from build123d import *

# Parameters (mm, degrees)
SKETCH1_R           = 2.1
SKETCH1_R_2         = 13
BOSS_EXTRUDE1_DEPTH = 0.4
BOSS_EXTRUDE2_DEPTH = 0.4


with BuildPart() as part:
    # Sketch1 → Boss-Extrude1 (new body)
    with BuildSketch(Plane(origin=(0, 0, 0), x_dir=(0, 1, 0), z_dir=(0, 0, 1))):
        with BuildLine():
            ThreePointArc((21.242857143, -3.31527079), (21.435617889, -1.662614121), (21.5, 0))
            ThreePointArc((21.5, 0), (21.435617889, 1.662614121), (21.242857143, 3.31527079))
            ThreePointArc((21.242857143, 3.31527079), (19.220493395, 4.694667451), (16.785714286, 4.948716593))
            ThreePointArc((16.785714286, 4.948716593), (12.374368671, 12.374368671), (4.948716593, 16.785714286))
            ThreePointArc((4.948716593, 16.785714286), (4.694667451, 19.220493395), (3.31527079, 21.242857143))
            ThreePointArc((3.31527079, 21.242857143), (0, 21.5), (-3.31527079, 21.242857143))
            ThreePointArc((-3.31527079, 21.242857143), (-4.694667451, 19.220493395), (-4.948716593, 16.785714286))
            ThreePointArc((-4.948716593, 16.785714286), (-12.374368671, 12.374368671), (-16.785714286, 4.948716593))
            ThreePointArc((-16.785714286, 4.948716593), (-19.220493395, 4.694667451), (-21.242857143, 3.31527079))
            ThreePointArc((-21.242857143, 3.31527079), (-21.5, 0), (-21.242857143, -3.31527079))
            ThreePointArc((-21.242857143, -3.31527079), (-19.220493395, -4.694667451), (-16.785714286, -4.948716593))
            ThreePointArc((-16.785714286, -4.948716593), (-12.374368671, -12.374368671), (-4.948716593, -16.785714286))
            ThreePointArc((-4.948716593, -16.785714286), (-4.694667451, -19.220493395), (-3.31527079, -21.242857143))
            ThreePointArc((-3.31527079, -21.242857143), (0, -21.5), (3.31527079, -21.242857143))
            ThreePointArc((3.31527079, -21.242857143), (4.694667451, -19.220493395), (4.948716593, -16.785714286))
            ThreePointArc((4.948716593, -16.785714286), (12.374368671, -12.374368671), (16.785714286, -4.948716593))
            ThreePointArc((16.785714286, -4.948716593), (19.220493395, -4.694667451), (21.242857143, -3.31527079))
        make_face()
        with Locations((0, -17.5)):
            Circle(SKETCH1_R, mode=Mode.SUBTRACT)
        Circle(SKETCH1_R_2, mode=Mode.SUBTRACT)
        with Locations((17.5, 0)):
            Circle(SKETCH1_R, mode=Mode.SUBTRACT)
        with Locations((-17.5, 0)):
            Circle(SKETCH1_R, mode=Mode.SUBTRACT)
        with Locations((0, 17.5)):
            Circle(SKETCH1_R, mode=Mode.SUBTRACT)
    extrude(amount=BOSS_EXTRUDE1_DEPTH)

    # Sketch1_4 → Boss-Extrude2 (add)
    with BuildSketch(Plane(origin=(0, 0, 0), x_dir=(0, 1, 0), z_dir=(0, 0, 1))):
        with BuildLine():
            ThreePointArc((-21.242857143, -3.31527079), (-15.202795796, -15.202795796), (-3.31527079, -21.242857143))
            ThreePointArc((-3.31527079, -21.242857143), (-4.694667451, -19.220493395), (-4.948716593, -16.785714286))
            ThreePointArc((-4.948716593, -16.785714286), (-12.374368671, -12.374368671), (-16.785714286, -4.948716593))
            ThreePointArc((-16.785714286, -4.948716593), (-19.220493395, -4.694667451), (-21.242857143, -3.31527079))
        make_face()
        with BuildLine():
            ThreePointArc((-4.948716593, 16.785714286), (-4.694667451, 19.220493395), (-3.31527079, 21.242857143))
            ThreePointArc((-3.31527079, 21.242857143), (-15.202795796, 15.202795796), (-21.242857143, 3.31527079))
            ThreePointArc((-21.242857143, 3.31527079), (-19.220493395, 4.694667451), (-16.785714286, 4.948716593))
            ThreePointArc((-16.785714286, 4.948716593), (-12.374368671, 12.374368671), (-4.948716593, 16.785714286))
        make_face()
        with BuildLine():
            ThreePointArc((16.785714286, 4.948716593), (19.220493395, 4.694667451), (21.242857143, 3.31527079))
            ThreePointArc((21.242857143, 3.31527079), (15.202795796, 15.202795796), (3.31527079, 21.242857143))
            ThreePointArc((3.31527079, 21.242857143), (4.694667451, 19.220493395), (4.948716593, 16.785714286))
            ThreePointArc((4.948716593, 16.785714286), (12.374368671, 12.374368671), (16.785714286, 4.948716593))
        make_face()
        with BuildLine():
            ThreePointArc((3.31527079, -21.242857143), (15.202795796, -15.202795796), (21.242857143, -3.31527079))
            ThreePointArc((21.242857143, -3.31527079), (19.220493395, -4.694667451), (16.785714286, -4.948716593))
            ThreePointArc((16.785714286, -4.948716593), (12.374368671, -12.374368671), (4.948716593, -16.785714286))
            ThreePointArc((4.948716593, -16.785714286), (4.694667451, -19.220493395), (3.31527079, -21.242857143))
        make_face()
    extrude(amount=BOSS_EXTRUDE2_DEPTH)


solid = part.part
Can you work these out from the model? Positions are in its coordinate system, mm. Give positions to 0.01 mm unless a question says otherwise; leave off trailing zeros. Order: outer loops, then holes, each group sorted by start corner. A loop starts at its lowest first (then second) coordinate and runs counter-clockwise, first axis right, second up. Notation, with made-up numbers: M 37.5,6 L 41.5,6 A32 cw 41.5,37 Z; hole C 60,-22.5 d10. An arc over 180 degrees is marked long. Use one line per item in the form item = value.
Item 1: If we section it at A-A, the plane y = 0: Write out the boundary of the cut face in (x, z).
Values follow:
outline = M -21.5,0 L -19.6,0 L -19.6,0.4 L -21.5,0.4 Z; M -15.4,0 L -13,0 L -13,0.4 L -15.4,0.4 Z; M 13,0 L 15.4,0 L 15.4,0.4 L 13,0.4 Z; M 19.6,0 L 21.5,0 L 21.5,0.4 L 19.6,0.4 Z
Item 2: Thinking about a two-plate mould opening in X: for faces 1 (the flat face through (9.3, 9.3, 0.4)), 2 (the cylindrical face through (-0.631, 19.503, 0.197)), which applies, pulls with the +X half, pulls with the -X half, needs draft (parallel to the pull), parting line crosses it, or undercut?
Values follow:
face_1 = needs draft
face_2 = undercut
Item 3: If we section it at B-B, the plane x = -17.5: Write out the boundary of the cut face in (y, z), and give its area (3 significant figures).
Values follow:
outline = M -12.49,0 L -2.1,0 L -2.1,0.4 L -12.49,0.4 Z; M 2.1,0 L 12.49,0 L 12.49,0.4 L 2.1,0.4 Z
area = 8.31 mm^2
Item 4: If we section it at C-C, the plane z = 0.2: Write out the boundary of the cut face in (x, y).
Values follow:
outline = C 0,0 d43; hole C -17.5,0 d4.2; hole C 0,0 d26; hole C 0,-17.5 d4.2; hole C 0,17.5 d4.2; hole C 17.5,0 d4.2
Item 5: If I drill on line 1 along X through (y, z) = (0, 0.1); line 2 along Y through (x, z) = (-8, 0.1), over which ranges is the centre line in solid material (lowest first)? Write a range as [from, to].
Values follow:
line_1 = [-21.5, -19.6], [-15.4, -13], [13, 15.4], [19.6, 21.5]
line_2 = [-19.96, -10.25], [10.25, 19.96]
